Source: CAD feature listing. Evaluate the final solid. Frame: model axes, mm. A direction names the side the tool comes from. Give positions to 0.01 mm unless a question says otherwise; leave off trailing zeros. Loops run counter-clockwise (first coordinate to the right, second up) from the corner with the lowest first, then second, coordinate; pieces in that order, holes last. Notation, with made-up numbers: M -14,-22.75 L 10,-22.75 A35 cw 10,14.25 Z; hole C 20.5,65.25 d7. An arc over 180 degrees is marked long. Put each result on its own line as item: value.
Autodesk Inventor part; units mm, degrees
ref_plane "YZ Plane" through (0, 0, 0) normal (1, 0, 0) x (0, 1, 0)
ref_plane "XZ Plane" through (0, 0, 0) normal (0, 1, 0) x (-1, 0, 0)
ref_plane "XY Plane" through (0, 0, 0) normal (0, 0, 1) x (1, 0, 0)
sketch "草图1" plane through (0, 0, 0) normal (0, 0, 1) x (1, 0, 0)
  line L0 (24.9, 16.8) -> (24.9, 0)
  line L1 (24.9, 0) -> (24.9, -16.8)
  line L2 (24.9, 0) -> (41.7, 0) construction
  line L3 (24.9, -16.8) -> (21.24, -16.8)
  line L4 (24.9, 16.8) -> (21.24, 16.8)
  line L5 (-16.8, 24.9) -> (0, 24.9)
  line L6 (0, 24.9) -> (16.8, 24.9)
  line L7 (16.8, 24.9) -> (16.8, 21.24)
  line L8 (-16.8, 24.9) -> (-16.8, 21.24)
  line L9 (-24.9, -16.8) -> (-24.9, 0)
  line L10 (-24.9, 0) -> (-24.9, 16.8)
  line L11 (-24.9, 0) -> (-41.7, 0) construction
  line L12 (-24.9, 16.8) -> (-21.24, 16.8)
  line L13 (-24.9, -16.8) -> (-21.24, -16.8)
  line L14 (16.8, -24.9) -> (0, -24.9)
  line L15 (0, -24.9) -> (-16.8, -24.9)
  line L16 (-16.8, -24.9) -> (-16.8, -21.24)
  line L17 (16.8, -24.9) -> (16.8, -21.24)
  line L18 (-21.24, 16.8) -> (-16.8, 21.24)
  line L19 (16.8, 21.24) -> (21.24, 16.8)
  line L20 (21.24, -16.8) -> (16.8, -21.24)
  line L21 (-16.8, -21.24) -> (-21.24, -16.8)
  point P0 (0, 0)
extrude "拉伸1" add sketch "草图1" along normal blind 7
sketch "草图2" plane through (-16.8, 24.9, 0) normal (0, 1, 0) x (1, 0, 0)
  line L0 (0, -7) -> (33.6, -7)
  point P0 (16.8, -3.5)
hole "孔1" at (0, 24.9, 3.5) direction (0, -1, 0) diameter 2.97 end through all counterbore diameter 6 counterbore depth 3
sketch "草图3" plane through (-16.8, -24.9, 0) normal (0, -1, 0) x (1, 0, 0)
  point P0 (16.8, 3.5)
hole "孔2" at (0, -24.9, 3.5) direction (0, 1, 0) diameter 2.97 end through all counterbore diameter 6 counterbore depth 3
sketch "草图4" plane through (24.9, -16.8, 0) normal (1, 0, 0) x (0, 0, -1)
  point P0 (0, 16.8)
  point P1 (-3.5, 16.8)
hole "孔3" at (24.9, 0, 3.5) direction (-1, 0, 0) diameter 2.97 end through all counterbore diameter 6 counterbore depth 3
sketch "草图5" plane through (-24.9, -16.8, 0) normal (-1, 0, 0) x (0, 0, 1)
  point P0 (0, 16.8)
  point P1 (3.5, 16.8)
hole "孔4" at (-24.9, 0, 3.5) direction (1, 0, 0) diameter 2.97 end through all counterbore diameter 6 counterbore depth 3
sketch "草图6" plane through (0, 0, 0) normal (0, 0, -1) x (-1, 0, 0)
  point P0 (0, 0)
hole "孔5" at (0, 0, 0) direction (0, 0, 1) diameter 22 end through all
equation "\"d53\" = Thickness"
equation "\"BendRadius\" = Thickness"
equation "\"BendReliefWidth\" = Thickness"
equation "\"BendReliefDepth\" = 0.5 * Thickness"
equation "\"CornerReliefSize\" = 4 * Thickness"
equation "\"MinimumRemnant\" = 2 * Thickness"
equation "\"TransitionRadius\" = BendRadius"
equation "\"JacobiRadiusSize\" = BendRadius"
properties part number "LaserHolder_20mm"
1. Section query C-C (x = 7). Output: boundary loops of the cut face in (y, z).
Found:
outline: M -24.9,0 L -8.49,0 L -8.49,7 L -24.9,7 Z; M 8.49,0 L 24.9,0 L 24.9,7 L 8.49,7 Z
2. Contact query for flat-ended pins moving along their axis: P1, Ø1.8, axis at y = -22.5, z = 3.5, coming from the -X side; P2, Ø2.5, axis at y = 0, z = 3.5, coming from the -X side; P3, Ø3.5, axis at y = 0, z = 3.5, coming from the -X side; P4, Ø1.8, axis at x = -23, z = 2.5, coming from the +Y side. Output: stop coordinate, or through.
Found:
P1: x = -16.8
P2: through
P3: x = -21.9
P4: y = 16.8
3. Section query D-D (y = -14). Output: boundary loops of the cut face in (x, z) (3 decimals), plus the area to 3 significant figures.
Found:
outline: M -24.9,0 L 24.9,0 L 24.9,7 L -24.9,7 Z; hole C 0,3.5 d2.97
area: 342 mm^2
4. Access query for faces 4 (the flat face through (-21.9, 1, 2)), 5 (the flat face through (23, 16.8, 3)), 6 (the flat face through (-16.8, -23, 3)), 7 (the cylindrical face through (1.8, -23.4, 5.9)). Directions: +Z, -Z, +X, -X, +Y, -Y. A direction counts if a zero-diameter tool reaches every point of the face in a straight line with its end or side. Return the directions, or none.
Found:
face 4: -X
face 5: +Z, -Z, +X, +Y
face 6: +Z, -Z, -X, -Y
face 7: -Y
5. Section query A-A (y = 0). Output: boundary loops of the cut face in (x, z) (3 decimals).
Found:
outline: M -24.9,0 L -11,0 L -11,2.015 L -21.9,2.015 L -21.9,0.5 L -24.9,0.5 Z; M -24.9,6.5 L -21.9,6.5 L -21.9,4.985 L -11,4.985 L -11,7 L -24.9,7 Z; M 11,0 L 24.9,0 L 24.9,0.5 L 21.9,0.5 L 21.9,2.015 L 11,2.015 Z; M 11,4.985 L 21.9,4.985 L 21.9,6.5 L 24.9,6.5 L 24.9,7 L 11,7 Z
6. Draft query along Y for faces 1 (the flat face through (-16.8, 23, 3)), 2 (the flat face through (-23, 16.8, 3)), 3 (the flat face through (21.9, 1, 5)). Return one class per face: pulls with the +Y half, pulls with the -Y half, needs draft (parallel to the pull), parting line crosses it, or undercut.
Found:
face 1: needs draft
face 2: pulls with the +Y half
face 3: undercut
7. Material intervals for line 1 (Z direction, x = 0, y = -15) (3 decimals); line 2 (X direction, y = -24.05, z = 3.5); line 3 (Z direction, x = 23, y = 0), sorted ascending. Write a range as from..to.
Found:
line 1: 0..2.015, 4.985..7
line 2: -16.8..-3, 3..16.8
line 3: 0..0.5, 6.5..7
